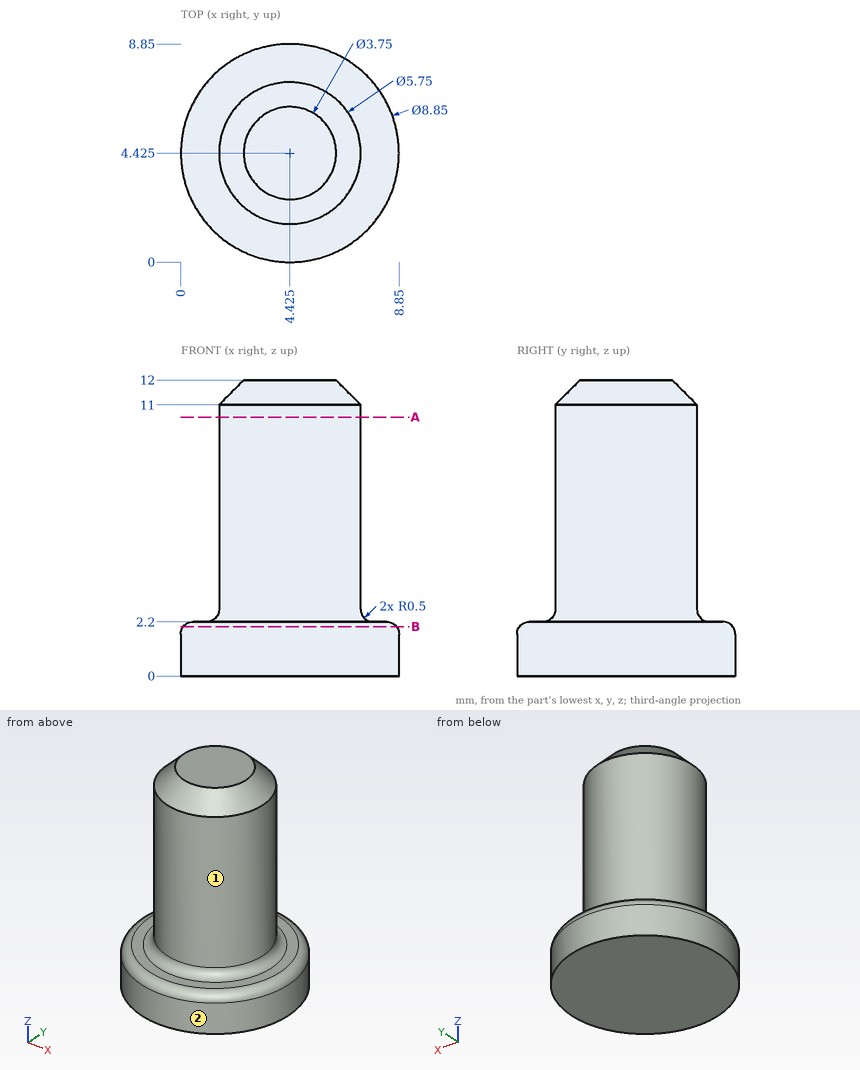
Answer from the drawing. Dimensions are ordinates in mm from the lowest x, y and z of the part. A direction names the side the tool comes from. Coordinates: 2 decimals unless noted, no trailing zeros. Loops run counter-clockwise (first coordinate to the right, second up) from the corner with the lowest first, then second, coordinate; pieces in that order, holes last. Notation, with made-up numbers: (1.25, 34.25) -> (46.25, 34.25) arc R26 cw to (46.25, 54.25) -> close; hole circle Ø4 at (-31, 7.5). An arc over 180 degrees is marked (long way). Return JSON: item names as keys, results as strings.
Item 1: Find section B-B (z = 2). Determine the outline of the cut face in (x, y) (3 decimals), plus the area to 3 significant figures.
Answers:
{"outline": "circle Ø8.65 at (4.425, 4.425)", "area": "58.8 mm2"}
Item 2: For the marked faces 1 and 2, determine the directions among +Z, -Z, +X, -X, +Y, -Y from which every point of the face is accessible in a straight line to the end or side of a thin tool.
Answers:
{"face 1": "+Z", "face 2": "+Z, -Z"}
Item 3: Flat-ended cylindrical pins translate along their axes: P1, Ø2, axis at x = 1.5, z = 7, coming from the -Y side; P2, Ø1.5, axis at x = 5.5, z = 5.5, coming from the +Y side; P3, Ø3, axis at x = 7, z = 2.5, coming from the +Y side. Find the tip coordinate at first contact, or state that the pin passes through.
Answers:
{"P1": "stops at y = 2.29", "P2": "stops at y = 7.28", "P3": "stops at y = 8.66"}
Item 4: Find the intervals of material crossed by probe 1 along Z at (x, y) = (1.5, 2); probe 2 along Y at (x, z) = (4, 6.5); probe 3 along X at (y, z) = (2, 3.5), in increasing order.
Answers:
{"probe 1": "z = 0 to 2.2", "probe 2": "y = 1.58 to 7.27", "probe 3": "x = 2.88 to 5.97"}
Item 5: Find section A-A (z = 10.5). Determine the outline of the cut face in (x, y) (3 decimals).
Answers:
{"outline": "circle Ø5.75 at (4.425, 4.425)"}
